The figure shows three views and two pictorial views of one solid part (mm, origin at its lowest corner). Answer the questions. A direction names the side the tool comes from. Round coordinates to 2 decimals unless told otherwise and drop trailing zeros. Order: outer loops, then holes, each group sorted by start corner. A loop starts at its lowest first (then second) coordinate and runs counter-clockwise, first axis right, second up. Notation, with made-up numbers: (-6.75, 35.5) -> (19.25, 35.5) arc R21 cw to (19.25, 55.5) -> close; hole circle Ø8 at (-39, 20). An arc over 180 degrees is marked (long way). Return JSON: item names as keys, results as strings. Group by question number.
(1) Determine the mould class of the marked faces 1, 2 and 3 for opening direction Z: +Z half, -Z half, draft (parallel to the pull), parting line (faces both ways), or undercut.
(2) The part is cut by section D-D (y = 17.5). Determine the outline of the cut face in (x, z) (1 decimal), plus the area to 3 significant figures.
(3) Each of these flat-tipped pins is pushed along its axis until it touches: pin 1 (10 mm diameter, centred on y = 18, z = 6, fed in from -X); pin 2 (1 mm diameter, centred on x = 33, z = 19.5, fed in from +Y). Where does it stop, or does it pass through?
(4) The part is cut by section B-B (z = 12.7). Count the separate pieces of the cut face and the enclosed holes in it, plus the area to 3 significant figures.
(5) Which of the six approach directions +Z, -Z, +X, -X, +Y, -Y give full straight-line access (tool end or side, diameter ignored) to the marked faces 4 and 5?
(6) The part is cut by section C-C (x = 19.05). Determine the outline of the cut face in (y, z).
(7) The part is cut by section A-A (y = 8.75). Determine the outline of the cut face in (x, z) (1 decimal).
(8) Consider line 1 (Z direction, x = 19.05, y = 1.45); line 2 (X direction, y = 8.75, z = 22.5) (1 decimal); line 3 (Y direction, x = 23, z = 11.25). Determine where each line is inside the solid, lowest interval first. Write a range as [from, to].
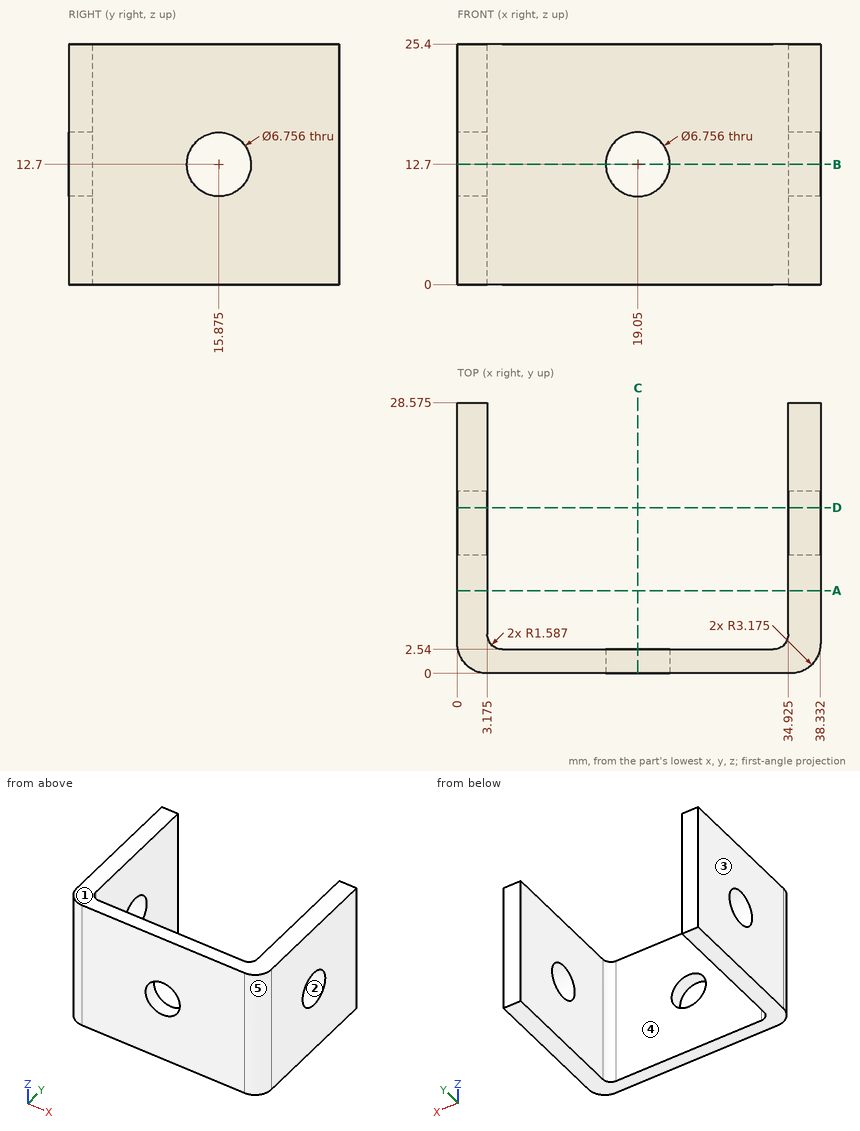
Answer below:
{
 "1": {"face 1": "+Z half", "face 2": "undercut", "face 3": "draft"},
 "2": {"outline": "(0, 0) -> (3.2, 0) -> (3.2, 9.7) -> (0, 9.7) -> close; (0, 15.7) -> (3.2, 15.7) -> (3.2, 25.4) -> (0, 25.4) -> close; (34.9, 0) -> (38.3, 0) -> (38.3, 9.7) -> (34.9, 9.7) -> close; (34.9, 15.7) -> (38.3, 15.7) -> (38.3, 25.4) -> (34.9, 25.4) -> close", "area": "128 mm²"},
 "3": {"pin 1": "stops at x = 0", "pin 2": "stops at y = 2.55"},
 "4": {"separate pieces": "4", "enclosed holes": "0", "area": "204 mm²"},
 "5": {"face 4": "+Z, -Z, +Y", "face 5": "+Z, -Z, +X, -Y"},
 "6": {"outline": "(0, 0) -> (2.54, 0) -> (2.54, 9.32) -> (0, 9.32) -> close; (0, 16.08) -> (2.54, 16.08) -> (2.54, 25.4) -> (0, 25.4) -> close"},
 "7": {"outline": "(0, 0) -> (3.2, 0) -> (3.2, 25.4) -> (0, 25.4) -> close; (34.9, 0) -> (38.3, 0) -> (38.3, 25.4) -> (34.9, 25.4) -> close"},
 "8": {"line 1": "z = [0, 9.32], [16.08, 25.4]", "line 2": "x = [0, 3.2], [34.9, 38.3]", "line 3": "y = [0, 2.54]"}
}
